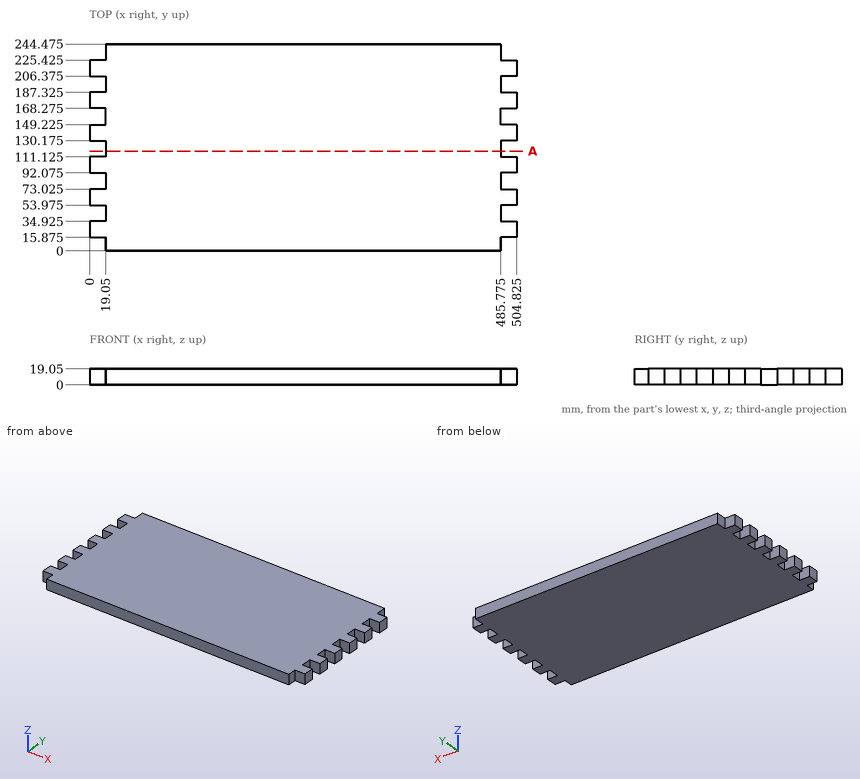
Answer from the drawing. Dimensions are ordinates in mm from the lowest x, y and z of the part. Coordinates: 2 decimals unless noted, no trailing zeros. Loops run counter-clockwise (first coordinate to the right, second up) from the corner with the lowest first, then second, coordinate; pieces in that order, holes last.
Q1. The part is cut by section A-A on y = 118. Write down the section's boundary in (x, z) (3 decimals), and give its area (3 significant figures).
Q2. Consider probe 1 along X at (y, z) = (226, 5.75) (3 decimals). Determine where the line is inside the solid, lowest interval first.
Q3. Each of these flat-tipped pins is pushed along its axis until it touches: pin 1 Ø5.5 at (x, z) = (492.5, 11) entering from +Y (3 decimals); pin 2 Ø5.5 at (y, z) = (83, 8) entering from -X; pin 3 Ø5.5 at (y, z) = (193.5, 7) entering from +X (3 decimals). Where does it stop, or does it pass through?
Results below:
1. outline: (19.05, 0) - (485.775, 0) - (485.775, 19.05) - (19.05, 19.05) - close
1. area: 8,890 mm2
2. probe 1: x = 19.05 to 485.775
3. pin 1: stops at y = 225.425
3. pin 2: stops at x = 19.05
3. pin 3: stops at x = 485.775
